For this review, take the finished solid that the model builds, in its own axes (mm). A direction names the side the tool comes from. Round coordinates to 2 decimals unless told otherwise and drop trailing zeros. Write each loop counter-clockwise with the first axis right and the second up, starting at its lowest first coordinate (ties: lowest second). Pieces come first, ordered by that corner, then holes.
from build123d import *

# Parameters (mm, degrees)
BOSS_EXTRUDE1_DEPTH = 30
BOSS_EXTRUDE2_DEPTH = 250
BOSS_EXTRUDE3_DEPTH = 8
BOSS_EXTRUDE4_DEPTH = 10
CHAMFER1_SIZE2      = 47.117047316
CHAMFER1_SIZE       = 20


with BuildPart() as part:
    # Sketch1 → Boss-Extrude1 (new body)
    with BuildSketch(Plane.XY):
        Polygon((0, 0), (21, 0), (21, -30), (29, -30), (29, 10), (-8, 10), (-8, -30), (0, -30), align=None)
    extrude(amount=BOSS_EXTRUDE1_DEPTH)

    # Sketch2 → Boss-Extrude2 (add)
    with BuildSketch(Plane.ZY.offset(8)):
        with BuildLine():
            Line((0, -22.811969958), (0, 3.313687916))
            ThreePointArc((0, 3.313687916), (15.101138891, 9.997881194), (30, 2.874204248))
            Line((30, 2.874204248), (30, -22.37248629))
            ThreePointArc((30, -22.37248629), (15.101138891, -29.496163235), (0, -22.811969958))
        make_face()
    extrude(amount=BOSS_EXTRUDE2_DEPTH)

    # Sketch3 → Boss-Extrude3 (add)
    with BuildSketch(Plane.ZY.offset(258)):
        with BuildLine():
            Line((30, -22.37248629), (30, 37.034794094))
            ThreePointArc((30, 37.034794094), (15, 43.247997529), (0, 37.034794094))
            Line((0, 37.034794094), (0, -22.811969958))
            ThreePointArc((0, -22.811969958), (15.101138891, -29.496163235), (30, -22.37248629))
        make_face()
    extrude(amount=BOSS_EXTRUDE3_DEPTH)

    # Sketch4 → Boss-Extrude4 (add)
    with BuildSketch(Plane.XY):
        Polygon((-84.478678947, -22.37248629), (0, -119.738410874), (0, -30), (-8, -30), (-8, -80), (-58, -22.37248629), align=None)
    extrude(amount=BOSS_EXTRUDE4_DEPTH)

    # Chamfer1
    chamfer1_edges = [part.edges().sort_by_distance(p)[0] for p in [
        (-4, -30, 10),
    ]]
    chamfer1_side = [part.faces().sort_by_distance(p)[0] for p in [
        (-4, -30, 10.4),
    ]]
    chamfer(chamfer1_edges, length=CHAMFER1_SIZE - 0.0001, length2=CHAMFER1_SIZE2 - 0.0001, reference=chamfer1_side[0])  # a hair under: the kernel refuses the full size


solid = part.part
(1) We need section B-B, the plane y = -45.5. Give the boundary of the cut face in (x, z).
Geometry check:
outline: (-64.41, 0) - (-37.93, 0) - (-37.93, 10) - (-64.41, 10) - close; (-8, 0) - (0, 0) - (0, 23.42) - (-8, 23.42) - close
(2) For pin 1 Ø8 at (y, z) = (-74.5, 18.5) entering from -X; pin 2 Ø2.5 at (x, z) = (25, 10) entering from -Y; pin 3 Ø3 at (x, z) = (-130.5, 25.5) entering from -Y; pin 4 Ø15 at (y, z) = (-68.5, 18) entering from +X, all flat-tipped, find the tip position at first contact; note any pin that passes through.
Geometry check:
pin 1: passes through
pin 2: stops at y = -30
pin 3: stops at y = -27.23
pin 4: stops at x = 0
(3) For faces 1 (the face through (11, 10, 15)), 2 (the face through (-8, 8, 26)), 3 (the face through (10, 0, 15)), 4 (the face through (25, -30, 15)), 5 (the face through (-8, 8, 3)), list the 3-axis set-ups (+Z, -Z, +X, -X, +Y, -Y) from which the entire face can be reached by the end or side of a thin tool; tool diameter is ignored.
Geometry check:
face 1: +Z, -Z, +X, +Y
face 2: +Z, +Y
face 3: +Z, -Z, -Y
face 4: +Z, -Z, +X, -Y
face 5: -Z, +Y
(4) Mouldability with a two-part tool opening along X and no side actions: class faces 6 (the face through (-107, -18, 0)), 7 (the face through (29, -10, 15)), 8 (the face through (-131, 10, 15)) as pulls with the +X half, pulls with the -X half, needs draft (parallel to the pull), parting line crosses it, or undercut.
Geometry check:
face 6: needs draft
face 7: pulls with the +X half
face 8: undercut
(5) We need section D-D, the plane y = 7. Give the boundary of the cut face in (x, z), and give its area (3 significant figures).
Geometry check:
outline: (-266, 0) - (-258, 0) - (-258, 4.35) - (-8, 4.35) - (-8, 0) - (29, 0) - (29, 30) - (-8, 30) - (-8, 25.28) - (-258, 25.28) - (-258, 30) - (-266, 30) - close
area: 6,580 mm2
(6) We need section C-C, the plane z = 6.5. Give the boundary of the cut face in (x, y), and give its area (3 significant figures).
Geometry check:
outline: (-266, -27.66) - (-79.89, -27.66) - (0, -119.74) - (0, 0) - (21, 0) - (21, -30) - (29, -30) - (29, 10) - (-8, 10) - (-8, 8.17) - (-258, 8.17) - (-258, 41.47) - (-266, 41.47) - close; hole (-53.41, -27.66) - (-8, -80) - (-8, -27.66) - close
area: 12,800 mm2
(7) We need section A-A, the plane x = -20. Give the boundary of the cut face in (y, z).
Geometry check:
outline: (-96.69, 0) - (-66.17, 0) - (-66.17, 10) - (-96.69, 10) - close; (-22.81, 0) - (3.31, 0) arc R19.75 ccw to (2.87, 30) - (-22.37, 30) arc R19.75 ccw to start
(8) For line 1 along X through (y, z) = (-19.5, 15); line 2 along Y through (x, z) = (13.5, 21); line 3 along X through (y, z) = (-71, 12), list the stretches that pass through material, from the lowest coordinate up.
Geometry check:
line 1: x = -266 to 0, 21 to 29
line 2: y = 0 to 10
line 3: x = -8 to 0
